from build123d import *

# Parameters (mm, degrees)
PAD002_DEPTH            = 0.4
SKETCH005_R             = 2
POCKET002_DEPTH         = 5
PAD003_DEPTH            = 3.85
POCKET003_DEPTH         = 4.251
POCKET004_DEPTH         = 3.45
FILLET003_R             = 0.7
FILLET004_R             = 0.5
FILLET005_R             = 1.1
FILLET006_R             = 0.9
BODY001_PLACEMENT_ANGLE = 180


with BuildPart() as part:
    # Sketch004 → Pad002 (new body)
    with BuildSketch(Plane.XY):
        with BuildLine():
            Line((-32.7, 6.275), (32.7, 6.275))
            ThreePointArc((34.7, 4.275), (34.114214, 5.689214), (32.7, 6.275))
            Line((34.7, 4.275), (34.7, -4.275))
            ThreePointArc((32.7, -6.275), (34.114214, -5.689214), (34.7, -4.275))
            Line((32.7, -6.275), (-32.7, -6.275))
            ThreePointArc((-34.7, -4.275), (-34.114214, -5.689214), (-32.7, -6.275))
            Line((-34.7, -4.275), (-34.7, 4.275))
            ThreePointArc((-32.7, 6.275), (-34.114214, 5.689214), (-34.7, 4.275))
        make_face()
    extrude(amount=PAD002_DEPTH)

    # Sketch005 (on Face10 of Pad002) → Pocket002 (cut)
    with BuildSketch(Plane.XY.offset(0.4)):
        with Locations((-31.755, 0)):
            Circle(SKETCH005_R)
        with Locations((31.755, 0)):
            Circle(SKETCH005_R)
    extrude(amount=-POCKET002_DEPTH, mode=Mode.SUBTRACT)

    # Sketch006 (on Face5 of Pocket002) → Pad003 (join)
    with BuildSketch(Plane.XY.offset(0.4)):
        with BuildLine():
            Line((-25.11, 5.4), (25.11, 5.4))
            ThreePointArc((28.852119, 0.939282), (28.021248, 4.04226), (25.11, 5.4))
            Line((28.852119, 0.939282), (28.287119, -2.260718))
            ThreePointArc((24.545, -5.4), (26.98726, -4.511248), (28.287119, -2.260718))
            Line((24.545, -5.4), (-24.545, -5.4))
            ThreePointArc((-28.287119, -2.260718), (-26.98726, -4.511248), (-24.545, -5.4))
            Line((-28.287119, -2.260718), (-28.852119, 0.939282))
            ThreePointArc((-25.11, 5.4), (-28.021248, 4.04226), (-28.852119, 0.939282))
        make_face()
    extrude(amount=PAD003_DEPTH)

    # Sketch007 (on Face21 of Pad003) → Pocket003 (cut, through all)
    with BuildSketch(Plane.XY.offset(4.25)):
        with BuildLine():
            Line((-25.11, 4.2), (25.11, 4.2))
            ThreePointArc((27.670397, 1.14793), (27.101906, 3.27102), (25.11, 4.2))
            Line((27.670397, 1.14793), (27.105397, -2.05207))
            ThreePointArc((24.545, -4.2), (26.21602, -3.591906), (27.105397, -2.05207))
            Line((24.545, -4.2), (-24.545, -4.2))
            ThreePointArc((-27.105397, -2.05207), (-26.21602, -3.591906), (-24.545, -4.2))
            Line((-27.105397, -2.05207), (-27.670397, 1.14793))
            ThreePointArc((-25.11, 4.2), (-27.101906, 3.27102), (-27.670397, 1.14793))
        make_face()
    extrude(amount=-POCKET003_DEPTH, mode=Mode.SUBTRACT)

    # Sketch008 (on Face4 of Pocket003) → Pocket004 (cut)
    with BuildSketch(Plane(origin=(0, 0, 0), x_dir=(1, 0, 0), z_dir=(0, 0, -1))):
        with BuildLine():
            Line((-24.545, 5), (24.545, 5))
            ThreePointArc((27.893211, 2.191169), (26.73018, 4.204801), (24.545, 5))
            Line((27.893211, 2.191169), (28.458211, -1.008831))
            ThreePointArc((25.11, -5), (27.714801, -3.78518), (28.458211, -1.008831))
            Line((25.11, -5), (-25.11, -5))
            ThreePointArc((-28.458211, -1.008831), (-27.714801, -3.78518), (-25.11, -5))
            Line((-28.458211, -1.008831), (-27.893211, 2.191169))
            ThreePointArc((-24.545, 5), (-26.73018, 4.204801), (-27.893211, 2.191169))
        make_face()
    extrude(amount=-POCKET004_DEPTH, mode=Mode.SUBTRACT)

    # Fillet003
    fillet003_edges = [part.edges().sort_by_distance(p)[0] for p in [
        (27.714801, 3.78518, 3.45),
    ]]
    fillet(fillet003_edges, radius=FILLET003_R)

    # Fillet004
    fillet004_edges = [part.edges().sort_by_distance(p)[0] for p in [
        (28.021248, 4.04226, 0.4),
    ]]
    fillet(fillet004_edges, radius=FILLET004_R)

    # Fillet005
    fillet005_edges = [part.edges().sort_by_distance(p)[0] for p in [
        (28.021248, 4.04226, 4.25),
    ]]
    fillet(fillet005_edges, radius=FILLET005_R)

    # Fillet006
    fillet006_edges = [part.edges().sort_by_distance(p)[0] for p in [
        (0, 5, 0),
    ]]
    fillet(fillet006_edges, radius=FILLET006_R)


with BuildPart() as part_1:
    # Body001 placement: moved
    add(part.part.rotate(Axis((0, 0, 0), (0, 1, 0)), BODY001_PLACEMENT_ANGLE))


solid = part_1.part
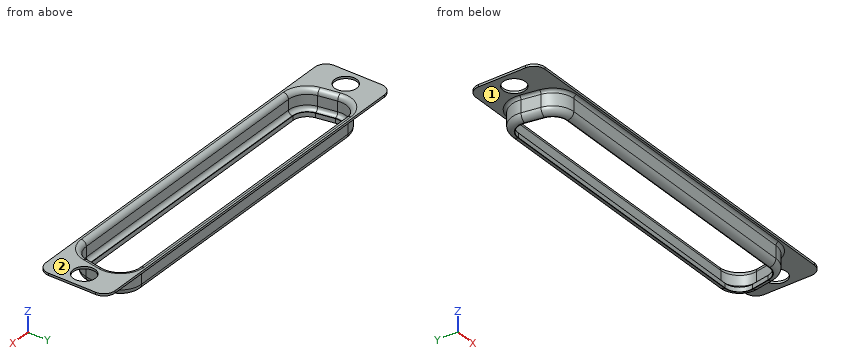
Geometry: final body of the model. Coordinates: model frame, mm. Face numbers are marked on the shaded views. A direction names the side the tool comes from. Round coordinates to 2 decimals unless told otherwise and drop trailing zeros. Loops run counter-clockwise (first coordinate to the right, second up) from the corner with the lowest first, then second, coordinate; pieces in that order, holes last.
Q1. Section B-B on z = -1.6. Return loops of the section in (x, y) (3 decimals).
Q2. Section A-A on x = -5.5. Return loops of the section in (y, z) (3 decimals).
Q3. Access query for the marked faces 1 and 2. Directions: +Z, -Z, +X, -X, +Y, -Y. A direction counts if a zero-diameter tool reaches every point of the face in a straight line with its end or side. Return the directions, or none.
Q4. Material intervals for L1, parallel to Y at x = 24.5, z = -2.35; L2, parallel to X at y = -2.25, z = -1.15; L3, parallel to Y at x = -12, z = -0.3 (3 decimals), sorted ascending.
Q5. Pin query (flat end, axial travel): P1, Ø5, axis at x = 13, y = 0.5, coming from the -Z side; P2, Ø0.7, axis at x = 11.5, z = -2, coming from the -Y side; P3, Ø6.5, axis at x = 31.755, y = 0, coming from the -Z side; P4, Ø7, axis at x = 10, y = 1, coming from the +Z side. Return the tip coordinate at first contact, or that it passes through.
Q6. Section C-C on y = 0. State how many separate pieces and enclosed holes the cut face has, plus the area to 3 significant figures.
Evaluation:
1. outline: (-28.852, 0.939) - (-28.287, -2.261) arc R3.8 ccw to (-24.545, -5.4) - (24.545, -5.4) arc R3.8 ccw to (28.287, -2.261) - (28.852, 0.939) arc R3.8 ccw to (25.11, 5.4) - (-25.11, 5.4) arc R3.8 ccw to start; hole (-28.458, 1.009) - (-27.893, -2.191) arc R3.4 ccw to (-24.545, -5) - (24.545, -5) arc R3.4 ccw to (27.893, -2.191) - (28.458, 1.009) arc R3.4 ccw to (25.11, 5) - (-25.11, 5) arc R3.4 ccw to start
2. outline: (-6.275, -0.4) - (-5.9, -0.4) arc R0.5 cw to (-5.4, -0.9) - (-5.4, -3.15) arc R1.1 ccw to (-4.3, -4.25) - (-4.2, -4.25) - (-4.2, -3.45) - (-4.3, -3.45) arc R0.7 cw to (-5, -2.75) - (-5, -0.9) arc R0.9 ccw to (-5.9, 0) - (-6.275, 0) - close; (4.2, -4.25) - (4.3, -4.25) arc R1.1 ccw to (5.4, -3.15) - (5.4, -0.9) arc R0.5 cw to (5.9, -0.4) - (6.275, -0.4) - (6.275, 0) - (5.9, 0) arc R0.9 ccw to (5, -0.9) - (5, -2.75) arc R0.7 cw to (4.3, -3.45) - (4.2, -3.45) - close
3. face 1: -Z
3. face 2: +Z, +X, -X, +Y, -Y
4. L1: y = -5.4 to -5, 5 to 5.4
4. L2: x = -28.29 to -27.88, 27.88 to 28.29
4. L3: y = -6.275 to -5.229, 5.229 to 6.275
5. P1: passes through
5. P2: stops at y = -5.4
5. P3: stops at z = -3.82
5. P4: stops at z = -3.42
6. separate pieces: 4
6. enclosed holes: 0
6. area: 5.81 mm2
